Verification items for the finished model (mm, model axes). A direction names the side the tool comes from. Give positions to 0.01 mm unless a question says otherwise; leave off trailing zeros. Order: outer loops, then holes, each group sorted by start corner. A loop starts at its lowest first (then second) coordinate and runs counter-clockwise, first axis right, second up. Notation, with made-up numbers: (81.5, 76) - (105.5, 76) arc R26 ccw to (105.5, 101) - close; hole circle Ø4 at (12.25, -38.75). An arc over 180 degrees is marked (long way). Answer as a JSON object with one key per item and string values.
```python
from build123d import *

# Parameters (mm, degrees)
SKETCH1_W           = 95
SKETCH1_H           = 51
BOSS_EXTRUDE1_DEPTH = 2
SKETCH2_W           = 95
SKETCH2_H           = 51
SKETCH2_W_2         = 90
SKETCH2_H_2         = 46
BOSS_EXTRUDE2_DEPTH = 6
SKETCH3_W           = 72
SKETCH3_H           = 28
CUT_EXTRUDE1_DEPTH  = 63.03729958
BOSS_EXTRUDE3_DEPTH = 4
SKETCH6_R           = 2.8
BOSS_EXTRUDE4_DEPTH = 3
SKETCH8_R           = 1.5
BOSS_EXTRUDE6_DEPTH = 15
FILLET1_R           = 1


with BuildPart() as part:
    # Sketch1 → Boss-Extrude1 (new body)
    with BuildSketch(Plane(origin=(0, 0, 0), x_dir=(1, 0, 0), z_dir=(0, 1, 0))):
        with Locations((-8.42936803, 0.663568773)):
            Rectangle(SKETCH1_W, SKETCH1_H)
    extrude(amount=BOSS_EXTRUDE1_DEPTH)

    # Sketch2 → Boss-Extrude2 (add)
    with BuildSketch(Plane(origin=(0, 2, 0), x_dir=(1, 0, 0), z_dir=(0, 1, 0))):
        with Locations((-8.42936803, 0.663568773)):
            Rectangle(SKETCH2_W, SKETCH2_H)
        with Locations((-8.42936803, 0.663568773)):
            Rectangle(SKETCH2_W_2, SKETCH2_H_2, mode=Mode.SUBTRACT)
    extrude(amount=BOSS_EXTRUDE2_DEPTH)

    # Sketch3 → Cut-Extrude1 (cut, through all)
    with BuildSketch(Plane(origin=(0, 2, 0), x_dir=(1, 0, 0), z_dir=(0, 1, 0))):
        with Locations((-8.42936803, 0.663568773)):
            Rectangle(SKETCH3_W, SKETCH3_H)
    extrude(amount=-CUT_EXTRUDE1_DEPTH, mode=Mode.SUBTRACT)

    # Sketch5 → Boss-Extrude3 (add)
    with BuildSketch(Plane.XZ):
        with BuildLine():
            Line((-49.67936803, -26.163568773), (-37.67936803, -26.163568773))
            Line((-37.67936803, -26.163568773), (-37.67936803, -36.163568773))
            ThreePointArc((-37.67936803, -36.163568773), (-43.67936803, -42.163568773), (-49.67936803, -36.163568773))
            Line((-49.67936803, -36.163568773), (-49.67936803, -26.163568773))
        make_face()
        with BuildLine():
            Line((-49.67936803, 24.836431227), (-49.67936803, 34.836431227))
            ThreePointArc((-49.67936803, 34.836431227), (-43.67936803, 40.836431227), (-37.67936803, 34.836431227))
            Line((-37.67936803, 34.836431227), (-37.67936803, 24.836431227))
            Line((-37.67936803, 24.836431227), (-49.67936803, 24.836431227))
        make_face()
        with BuildLine():
            Line((32.82063197, -26.163568773), (32.82063197, -36.163568773))
            ThreePointArc((32.82063197, -36.163568773), (26.82063197, -42.163568773), (20.82063197, -36.163568773))
            Line((20.82063197, -36.163568773), (20.82063197, -26.163568773))
            Line((20.82063197, -26.163568773), (32.82063197, -26.163568773))
        make_face()
        with BuildLine():
            Line((32.82063197, 24.836431227), (20.82063197, 24.836431227))
            Line((20.82063197, 24.836431227), (20.82063197, 34.836431227))
            ThreePointArc((20.82063197, 34.836431227), (26.82063197, 40.836431227), (32.82063197, 34.836431227))
            Line((32.82063197, 34.836431227), (32.82063197, 24.836431227))
        make_face()
    extrude(amount=-BOSS_EXTRUDE3_DEPTH)

    # Sketch6 → Boss-Extrude4 (add)
    with BuildSketch(Plane(origin=(0, 4, 0), x_dir=(1, 0, 0), z_dir=(0, 1, 0))):
        with Locations(Location((-43.67936803, 36.163568773, 0), (0, 0, 90))):
            Circle(SKETCH6_R)
        with Locations(Location((26.82063197, 36.163568773, 0), (0, 0, 270))):
            Circle(SKETCH6_R)
        with Locations(Location((26.82063197, -34.836431227, 0), (0, 0, 90))):
            Circle(SKETCH6_R)
        with Locations(Location((-43.67936803, -34.836431227, 0), (0, 0, 270))):
            Circle(SKETCH6_R)
    extrude(amount=BOSS_EXTRUDE4_DEPTH)

    # Sketch8 → Boss-Extrude6 (add)
    # profile 1 of 6: a face of its own
    with BuildSketch(Plane.XZ):
        with BuildLine():
            Line((-55.92936803, 24.836431227), (-58.92936803, 24.836431227))
            ThreePointArc((-58.92936803, 24.836431227), (-61.92936803, 21.836431227), (-58.92936803, 18.836431227))
            Line((-58.92936803, 18.836431227), (-55.92936803, 18.836431227))
            Line((-55.92936803, 18.836431227), (-55.92936803, 24.836431227))
        make_face()
        with Locations(Location((-58.92936803, 21.836431227, 0), (0, 0, 270))):
            Circle(SKETCH8_R, mode=Mode.SUBTRACT)
    # profile 2 of 6: a face of its own
    with BuildSketch(Plane.XZ):
        with BuildLine():
            Line((-5.42936803, -26.163568773), (-5.42936803, -29.163568773))
            ThreePointArc((-5.42936803, -29.163568773), (-8.42936803, -32.163568773), (-11.42936803, -29.163568773))
            Line((-11.42936803, -29.163568773), (-11.42936803, -26.163568773))
            Line((-11.42936803, -26.163568773), (-5.42936803, -26.163568773))
        make_face()
        with Locations(Location((-8.42936803, -29.163568773, 0), (0, 0, 90))):
            Circle(SKETCH8_R, mode=Mode.SUBTRACT)
    # profile 3 of 6: a face of its own
    with BuildSketch(Plane.XZ):
        with BuildLine():
            Line((-55.92936803, -20.163568773), (-58.92936803, -20.163568773))
            ThreePointArc((-58.92936803, -20.163568773), (-61.92936803, -23.163568773), (-58.92936803, -26.163568773))
            Line((-58.92936803, -26.163568773), (-55.92936803, -26.163568773))
            Line((-55.92936803, -26.163568773), (-55.92936803, -20.163568773))
        make_face()
        with Locations(Location((-58.92936803, -23.163568773, 0), (0, 0, 90))):
            Circle(SKETCH8_R, mode=Mode.SUBTRACT)
    # profile 4 of 6: a face of its own
    with BuildSketch(Plane.XZ):
        with BuildLine():
            Line((39.07063197, -26.163568773), (42.07063197, -26.163568773))
            ThreePointArc((42.07063197, -26.163568773), (45.07063197, -23.163568773), (42.07063197, -20.163568773))
            Line((42.07063197, -20.163568773), (39.07063197, -20.163568773))
            Line((39.07063197, -20.163568773), (39.07063197, -26.163568773))
        make_face()
        with Locations(Location((42.07063197, -23.163568773, 0), (0, 0, 270))):
            Circle(SKETCH8_R, mode=Mode.SUBTRACT)
    # profile 5 of 6: a face of its own
    with BuildSketch(Plane.XZ):
        with BuildLine():
            Line((39.07063197, 18.836431227), (42.07063197, 18.836431227))
            ThreePointArc((42.07063197, 18.836431227), (45.07063197, 21.836431227), (42.07063197, 24.836431227))
            Line((42.07063197, 24.836431227), (39.07063197, 24.836431227))
            Line((39.07063197, 24.836431227), (39.07063197, 18.836431227))
        make_face()
        with Locations(Location((42.07063197, 21.836431227, 0), (0, 0, 90))):
            Circle(SKETCH8_R, mode=Mode.SUBTRACT)
    # profile 6 of 6: a face of its own
    with BuildSketch(Plane.XZ):
        with BuildLine():
            Line((-11.42936803, 24.836431227), (-5.42936803, 24.836431227))
            Line((-5.42936803, 24.836431227), (-5.42936803, 27.836431227))
            ThreePointArc((-5.42936803, 27.836431227), (-8.42936803, 30.836431227), (-11.42936803, 27.836431227))
            Line((-11.42936803, 27.836431227), (-11.42936803, 24.836431227))
        make_face()
        with Locations(Location((-8.42936803, 27.836431227, 0), (0, 0, 270))):
            Circle(SKETCH8_R, mode=Mode.SUBTRACT)
    extrude(amount=-BOSS_EXTRUDE6_DEPTH)

    # Fillet1
    fillet1_edges = [part.edges().sort_by_distance(p)[0] for p in [
        (-44.42936803, 1, 13.336431227),
        (-44.42936803, 1, -14.663568773),
        (27.57063197, 1, -14.663568773),
        (27.57063197, 1, 13.336431227),
        (-49.67936803, 2, -26.163568773),
        (-37.67936803, 2, -26.163568773),
        (-37.67936803, 2, 24.836431227),
        (-49.67936803, 2, 24.836431227),
        (20.82063197, 2, -26.163568773),
        (32.82063197, 2, -26.163568773),
        (32.82063197, 2, 24.836431227),
        (20.82063197, 2, 24.836431227),
    ]]
    fillet(fillet1_edges, radius=FILLET1_R)


solid = part.part
```
(1) Material ranges on line 1 along X through (y, z) = (6.25, -23); line 2 along Z through (x, y) = (13, 7.5); line 3 along X through (y, z) = (7, 9.5), recorded low to high. Write a range as [from, to].
Computed values:
{"line 1": "x = [-61.92, -60.42], [-57.44, -53.43], [36.57, 40.58], [43.56, 45.07]", "line 2": "z = [-26.16, -23.66], [22.34, 24.84]", "line 3": "x = [-55.93, -53.43], [36.57, 39.07]"}
(2) Section check B-B (z = -10). Record the cut outline in (x, y), then the cut area to 3 significant figures.
Computed values:
{"outline": "(-55.93, 0) - (-44.43, 0) - (-44.43, 2) - (-53.43, 2) - (-53.43, 8) - (-55.93, 8) - close; (27.57, 0) - (39.07, 0) - (39.07, 8) - (36.57, 8) - (36.57, 2) - (27.57, 2) - close", "area": "76.0 mm²"}
(3) Section check C-C (z = 17). Record the cut outline in (x, y), then the cut area to 3 significant figures.
Computed values:
{"outline": "(-55.93, 0) - (39.07, 0) - (39.07, 8) - (36.57, 8) - (36.57, 2) - (-53.43, 2) - (-53.43, 8) - (-55.93, 8) - close", "area": "220 mm²"}
(4) Access from +Z, -Z, +X, -X, +Y, -Y to the whole of each face (thin tool, end or side, straight path). Record for faces 1 (the flat face through (39.071, 4, 0)), 2 (the flat face through (-57, 7, -20.164)), 3 (the cylindrical face through (-46.456, 5.479, -35.799)), 4 (the flat face through (-44, 7, -36)), 5 (the flat face through (-5.429, 7, -28)).
Computed values:
{"face 1": "+X, +Y, -Y", "face 2": "-X, +Y, -Y", "face 3": "+Y", "face 4": "-Z, +X, -X, +Y", "face 5": "-Z, +Y, -Y"}
(5) Release check for a two-part mould opening along Z. For faces 6 (the flat face through (40.7, 15, -24.5)), 7 (the cylindrical face through (45.07, 7.4, -23.23)), 8 (the cylindrical face through (-43.811, 1.972, 40.835)) record: pulls with the +Z half, pulls with the -Z half, needs draft (parallel to the pull), parting line crosses it, or undercut.
Computed values:
{"face 6": "needs draft", "face 7": "undercut", "face 8": "pulls with the +Z half"}
(6) Gauge pin test, flat ends, axial feed: pin 1 Ø1.5 at (x, y) = (25, 3) entering from +Z; pin 2 Ø5 at (x, y) = (-9, 12) entering from +Z; pin 3 Ø2.5 at (x, y) = (-57.5, 5.5) entering from +Z; pin 4 Ø2 at (x, z) = (-7.5, 10.5) entering from -Y. Record the tip position at first contact, or that the pin passes through.
Computed values:
{"pin 1": "stops at z = 40.74", "pin 2": "stops at z = 30.84", "pin 3": "stops at z = 24.84", "pin 4": "passes through"}
(7) Section check A-A (x = -24.5). Record the cut outline in (y, z).
Computed values:
{"outline": "(0, -26.16) - (8, -26.16) - (8, -23.66) - (2, -23.66) - (2, -14.66) - (0, -14.66) - close; (0, 13.34) - (2, 13.34) - (2, 22.34) - (8, 22.34) - (8, 24.84) - (0, 24.84) - close"}
